from build123d import *

# Parameters (mm, degrees)
EXTRUDE_1_DEPTH          = 9.5
EXTRUDE_1_DEPTH_BACK     = 9.5
SKETCH_1_R               = 4.5
CUT_EXTRUDE_1_DEPTH      = 7
CUT_EXTRUDE_1_DEPTH_BACK = 7
SKETCH_2_R               = 5.5
CUT_EXTRUDE_2_DEPTH      = 17.718253497
CUT_EXTRUDE_2_DEPTH_BACK = 17.718253497
SKETCH_3_R               = 1.5
CUT_EXTRUDE_3_DEPTH      = 7.5
CUT_EXTRUDE_3_DEPTH_BACK = 7.5
SKETCH_4_R               = 5.5
SKETCH_4_R_2             = 2.5
SKETCH_5_R               = 1.75
CUT_EXTRUDE_4_DEPTH      = 2


with BuildPart() as part:
    # Sketch 1 → Extrude 1 (new, two sides: drawn at the far end of the back side and taken through both)
    with BuildSketch(Plane(origin=(0, 0, 0), x_dir=(0, 0, -1), z_dir=(1, 0, 0)).offset(-EXTRUDE_1_DEPTH_BACK)):
        Circle(SKETCH_1_R)
        with BuildLine():
            Line((13, 4.5), (0, 4.5))
            ThreePointArc((0, 4.5), (3.181980515, 3.181980515), (4.5, 0))
            ThreePointArc((4.5, 0), (3.181980515, -3.181980515), (0, -4.5))
            Line((0, -4.5), (13, -4.5))
            Line((13, -4.5), (13, 4.5))
        make_face()
    extrude(amount=EXTRUDE_1_DEPTH + EXTRUDE_1_DEPTH_BACK)

    # Sketch 2 → Cut-Extrude 1 (cut, two sides: drawn at the far end of the back side and taken through both)
    with BuildSketch(Plane(origin=(0, 0, 0), x_dir=(0, 0, -1), z_dir=(1, 0, 0)).offset(-CUT_EXTRUDE_1_DEPTH_BACK)):
        Circle(SKETCH_2_R)
    extrude(amount=CUT_EXTRUDE_1_DEPTH + CUT_EXTRUDE_1_DEPTH_BACK, mode=Mode.SUBTRACT)

    # Sketch 3 → Cut-Extrude 2 (cut, two sides: drawn at the far end of the back side and taken through both)
    with BuildSketch(Plane(origin=(0, 0, 0), x_dir=(0, 0, -1), z_dir=(1, 0, 0)).offset(-CUT_EXTRUDE_2_DEPTH_BACK)):
        Circle(SKETCH_3_R)
    extrude(amount=CUT_EXTRUDE_2_DEPTH + CUT_EXTRUDE_2_DEPTH_BACK, mode=Mode.SUBTRACT)

    # Sketch 4 → Cut-Extrude 3 (cut, two sides: drawn at the far end of the back side and taken through both)
    with BuildSketch(Plane(origin=(0, 0, 0), x_dir=(0, 0, -1), z_dir=(1, 0, 0)).offset(-CUT_EXTRUDE_3_DEPTH_BACK)):
        Circle(SKETCH_4_R)
        Circle(SKETCH_4_R_2, mode=Mode.SUBTRACT)
    extrude(amount=CUT_EXTRUDE_3_DEPTH + CUT_EXTRUDE_3_DEPTH_BACK, mode=Mode.SUBTRACT)

    # Sketch 5 → Cut-Extrude 4 (cut)
    with BuildSketch(Plane(origin=(0, 0, -13), x_dir=(-1, 0, 0), z_dir=(0, 0, -1))):
        Circle(SKETCH_5_R)
    extrude(amount=-CUT_EXTRUDE_4_DEPTH, mode=Mode.SUBTRACT)


solid = part.part
The model under review builds one solid part; all positions refer to its coordinate system, in mm. A direction names the side the tool comes from. Coordinates: 2 decimals unless noted, no trailing zeros. Loops run counter-clockwise (first coordinate to the right, second up) from the corner with the lowest first, then second, coordinate; pieces in that order, holes last. Notation, with made-up numbers: M 2,0 L 61,0 A11 cw 61,11 Z; hole C -33.75,-33.75 d5. An arc over 180 degrees is marked long. Put each result on its own line as item: value. Start each with the question number.
Q1. Add section B-B (z = -11.5). Write out the cut boundary in (x, y).
Q2. Add section D-D (z = -4.5). Write out the cut boundary in (x, y), and give its area (3 significant figures).
Q3. Clearance check with flat-ended pins moving along their axes: pin 1 (5 mm diameter, centred on x = -1, z = 0, fed in from -Y); pin 2 (4 mm diameter, centred on y = 0.5, z = 1, fed in from -X); pin 3 (1.8 mm diameter, centred on x = 0, y = 0, fed in from -Z); pin 4 (2 mm diameter, centred on x = -6, y = 3, fed in from +Z). State where each tip first meets the part, or that it passes through.
Q4. The part is to be moulded in two halves that separate along X. For faces 4 (the flat face through (0, 4.5, -8)), 5 (the flat face through (-7, 0, -2)), 6 (the flat face through (-9.5, 0, -4)), 7 (the flat face through (-7.5, 0, -3)), say which applies: +X half, -X half, draft (parallel to the pull), parting line (faces both ways), or undercut.
Q5. Add section C-C (x = -4.5). Write out the cut boundary in (y, z).
Q6. For faces 1 (the flat face through (7, 0, -2)), 2 (the cylindrical face through (-7.25, -2.44, 0.54)), 3 (the flat face through (0, 0, -11)), list the 3-axis set-ups (+Z, -Z, +X, -X, +Y, -Y) from which the entire face can be reached by the end or side of a thin tool; tool diameter is ignored.
Q7. Add section A-A (y = -0.75). Write out the cut boundary in (x, z).
Q8. Wall thickness on line 1 (X direction, y = -2, z = 1.75); line 2 (Z direction, x = 8.3, y = 0); line 3 (X direction, y = 2, z = 0.75): over which ranges is each line inside the solid? List them lowest first.
Answers:
1. outline: M -9.5,-4.5 L 9.5,-4.5 L 9.5,4.5 L -9.5,4.5 Z; hole C 0,0 d3.5
2. outline: M -9.5,-4.5 L 9.5,-4.5 L 9.5,4.5 L -9.5,4.5 Z; hole M -7.5,-3.16 L 7.5,-3.16 L 7.5,3.16 L -7.5,3.16 Z
2. area: 76.1 mm^2
3. pin 1: passes through
3. pin 2: stops at x = -9.5
3. pin 3: stops at z = -11
3. pin 4: stops at z = -3.77
4. face 4: draft
4. face 5: undercut
4. face 6: -X half
4. face 7: undercut
5. outline: M -4.5,-13 L 4.5,-13 L 4.5,-3.16 A5.5 cw -4.5,-3.16 Z
6. face 1: +Z, +Y, -Y
6. face 2: none
6. face 3: -Z
7. outline: M -9.5,-13 L -1.58,-13 L -1.58,-11 L 1.58,-11 L 1.58,-13 L 9.5,-13 L 9.5,-1.3 L 7,-1.3 L 7,-2.38 L 7.5,-2.38 L 7.5,-5.45 L -7.5,-5.45 L -7.5,-2.38 L -7,-2.38 L -7,-1.3 L -9.5,-1.3 Z; M -9.5,1.3 L -7,1.3 L -7,2.38 L -7.5,2.38 L -7.5,4.44 L -9.5,4.44 Z; M 7,1.3 L 9.5,1.3 L 9.5,4.44 L 7.5,4.44 L 7.5,2.38 L 7,2.38 Z
8. line 1: x = -9.5 to -7.5, 7.5 to 9.5
8. line 2: z = -13 to -1.5, 1.5 to 4.5
8. line 3: x = -9.5 to -7, 7 to 9.5
